The model under review builds one solid part; all positions refer to its coordinate system, in mm. Face numbers are marked on the shaded views. A direction names the side the tool comes from. Round coordinates to 2 decimals unless told otherwise and drop trailing zeros. Loops run counter-clockwise (first coordinate to the right, second up) from the corner with the lowest first, then second, coordinate; pieces in that order, holes last. Notation, with made-up numbers: (40.5, -16) -> (91.5, -16) arc R13 ccw to (91.5, -4) -> close; hole circle Ø4 at (51, 13). An arc over 180 degrees is marked (long way). Use a Markdown table: item, result. Add a question column.
1) For the marked faces 1 and 2, list the 3-axis set-ups (+Z, -Z, +X, -X, +Y, -Y) from which the entire face can be reached by the end or side of a thin tool; tool diameter is ignored.
2) Insertion check: pin 1 (8 mm diameter, centred on x = 32, z = 12, fed in from +Y); pin 2 (17 mm diameter, centred on x = 28.5, y = -14.5, fed in from +Z); pin 3 (12 mm diameter, centred on x = -12.5, z = 11.5, fed in from +Y) (3 decimals). Each pin has a flat end and moves straight along its axis. Give the tip position at first contact, or say it passes through.
3) Consider section A-A on z = 23. Give the boundary of the cut face in (x, y), plus the area to 3 significant figures.
4) Consider section D-D on z = 11. Give the boundary of the cut face in (x, y).
5) Wall thickness on probe 1 along X at (y, z) = (-17, 2); probe 2 along Y at (x, z) = (0, 2.15); probe 3 along Z at (x, y) = (-3.5, -5): over which ranges is each line inside the solid? List them lowest first.
6) Consider section B-B on x = -12. Give the boundary of the cut face in (y, z).
7) Consider section C-C on y = -34. Give the boundary of the cut face in (x, z).
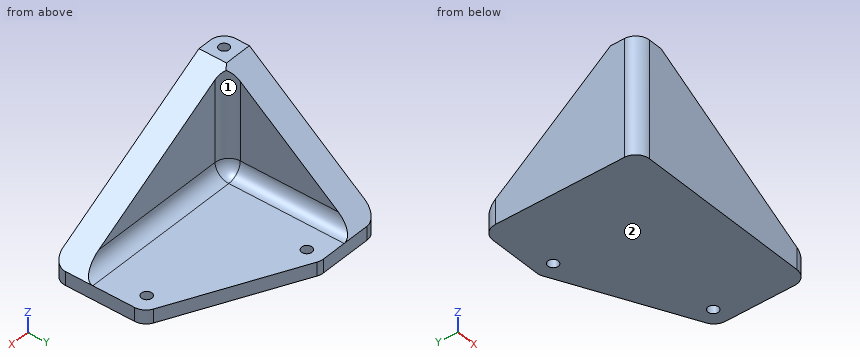
Autodesk Inventor part; units mm, degrees
ref_plane "YZ Plane" through (0, 0, 0) normal (1, 0, 0) x (0, 1, 0)
ref_plane "XZ Plane" through (0, 0, 0) normal (0, 1, 0) x (-1, 0, 0)
ref_plane "XY Plane" through (0, 0, 0) normal (0, 0, 1) x (1, 0, 0)
sketch "Sketch1" plane through (0, 0, 0) normal (0, 0, 1) x (1, 0, 0)
  line L0 (-19, 5) -> (40.5, 5)
  line L1 (40.5, 5) -> (40.5, -40.5)
  line L2 (40.5, -40.5) -> (-19, -40.5)
  line L3 (-19, -40.5) -> (-19, 5)
  line L4 (1.1354, 5) -> (40.5, -13.8506)
  line L5 (35.5, -17) -> (0, 0) construction
  point P0 (-15, -36.5)
  dimension "d0" = 35.5
  dimension "d1" = 17
  dimension "d2" = 50.5
  dimension "d3" = 19.5
  dimension "d4" = 5
  dimension "d5" = 5
  dimension "d6" = 4
  dimension "d7" = 4
  dimension "d31" = 5
extrude "Extrusion1" add sketch "Sketch1" along normal blind 4 contours L0 L4 L1 L2 L3
hole "Hole1" at (35.5, -17, 0) at (0, 0, 0) direction (0, 0, 1) diameter 3 depth 20
sketch "Sketch2" plane through (-19, -40.5, 0) normal (0, -1, 0) x (1, 0, 0)
  line L0 (0, 0) -> (59.5, 0)
  line L1 (59.5, 0) -> (59.5, 4)
  line L2 (0, 4) -> (59.5, 4)
  line L3 (0, 0) -> (0, 4)
  line L4 (0, 4) -> (0, 34)
  line L5 (0, 34) -> (8, 34)
  line L6 (8, 34) -> (59.5, 4)
  point P0 (19, 0)
  dimension "d17" = 34
  dimension "d18" = 8
extrude "Extrusion2" add sketch "Sketch2" against normal blind 8 contours L4 L5 L6 L2
sketch "Sketch3" plane through (-19, -40.5, 0) normal (-1, 0, 0) x (0, 0, 1)
  line L0 (0, 45.5) -> (0, 0)
  line L1 (0, 0) -> (34, 0)
  line L2 (34, 0) -> (34, 8)
  line L3 (4, 8) -> (34, 8)
  line L4 (4, 45.5) -> (4, 8)
  line L5 (0, 45.5) -> (4, 45.5)
  line L6 (34, 8) -> (4, 45.5)
  point P0 (0, 40.5)
extrude "Extrusion3" add sketch "Sketch3" against normal blind 8 contours L6 L3 L4
fillet "Fillet1" radius 4 8 edges at (-11, -13.75, 4) (14.75, -32.5, 4) (-11, -32.5, 19) (40.5, -40.5, 2) (-19, 5, 2) (1.1354, 5, 2) (40.5, -13.8506, 2) (-19, -40.5, 17)
sketch "Sketch4" plane through (-19, -40.5, 34) normal (0, 0, 1) x (1, 0, 0)
  line L0 (8, 0) -> (4, 0)
  line L1 (8, 0) -> (8, 8)
  line L2 (0, 8) -> (8, 8)
  line L3 (0, 4) -> (0, 8)
  arc A0 (0, 4) -> (4, 0) centre (4, 4) ccw
  point P0 (19, 40.5)
  point P1 (4, 4)
hole "Hole2" at (-15, -36.5, 34) direction (0, 0, -1) diameter 2.9 depth 20
equation "\"d5\" = d4"
equation "\"d23\" = d7"
properties part number "FrontLevelBlock" material "ABS Plastic"
Result set:
| question | item | result |
|---|---|---|
| 1 | face 1 | +Z, +X, +Y |
| 1 | face 2 | -Z, +X, -X, +Y, -Y |
| 2 | pin 1 | y = -32.5 |
| 2 | pin 2 | z = 4 |
| 2 | pin 3 | y = 3.125 |
| 3 | outline | (-19, -36.5) arc R4 ccw to (-15, -40.5) -> (7.88, -40.5) -> (7.88, -32.5) -> (-7, -32.5) arc R4 cw to (-11, -28.5) -> (-11, -18.75) -> (-19, -18.75) -> close; hole circle Ø2.9 at (-15, -36.5) |
| 3 | area | 318 mm2 |
| 4 | outline | (-19, -36.5) arc R4 ccw to (-15, -40.5) -> (28.48, -40.5) -> (28.48, -32.5) -> (-7, -32.5) arc R4 cw to (-11, -28.5) -> (-11, -3.75) -> (-19, -3.75) -> close |
| 5 | probe 1 | -19 to 34, 37 to 40.5 |
| 5 | probe 2 | -40.5 to -1.5, 1.5 to 5 |
| 5 | probe 3 | 0 to 4 |
| 6 | outline | (-40.5, 0) -> (5, 0) -> (5, 4) -> (-32.5, 34) -> (-40.5, 34) -> close |
| 7 | outline | (-19, 0) -> (40.5, 0) -> (40.5, 4) -> (-11, 34) -> (-19, 34) -> close |
